Geometry: final body of the model. Coordinates: model frame, mm. Coordinates: 2 decimals unless noted, no trailing zeros. Write each loop counter-clockwise with the first axis right and the second up, starting at its lowest first coordinate (ties: lowest second). Pieces come first, ordered by that corner, then holes. Notation, with made-up numbers: (-2, 13.25) -> (9, 13.25) arc R17 cw to (9, 40.25) -> close; hole circle Ø9 at (-13, 76.25). An arc over 180 degrees is marked (long way). Answer as a JSON object with one key per item and string values. Group by question number.
```python
from build123d import *

# Parameters (mm, degrees)
F1_DEPTH = 1.7
F2_R     = 3
F3_W     = 62.5
F3_H     = 32
F4_DEPTH = 1.701
F5_R     = 5


with BuildPart() as f1:
    # F0 (on Top) → F1 (new body)
    with BuildSketch(Plane.XY):
        Polygon((100.0762677759, 54.24722471), (-84.9237322241, 54.24722471), (-84.9237322241, 39.24722471), (-72.9237322241, 39.24722471), (-72.9237322241, 36.24722471), (-72.9237322241, -37.75277529), (-72.9237322241, -40.75277529), (-84.9237322241, -40.75277529), (-84.9237322241, -55.75277529), (100.0762677759, -55.75277529), (100.0762677759, -40.75277529), (88.0762677759, -37.75277529), (88.0762677759, 36.24722471), (88.0762677759, 39.24722471), (100.0762677759, 39.24722471), align=None)
        Polygon((88.0762677759, 36.24722471), (100.0762677759, 39.24722471), (88.0762677759, 39.24722471), align=None)
        Polygon((-72.9237322241, 39.24722471), (-84.9237322241, 39.24722471), (-72.9237322241, 36.24722471), align=None)
        Polygon((-72.9237322241, -40.75277529), (-72.9237322241, -37.75277529), (-84.9237322241, -40.75277529), align=None)
    extrude(amount=F1_DEPTH)

    # F2
    f2_edges = [f1.edges().sort_by_distance(p)[0] for p in [
        (-72.923732, -37.752775, 0.85),
        (-72.923732, 36.247225, 0.85),
        (-84.923732, 39.247225, 0.85),
        (-84.923732, -40.752775, 0.85),
        (88.076268, 36.247225, 0.85),
        (100.076268, 39.247225, 0.85),
        (-84.923732, -55.752775, 0.85),
        (-84.923732, 54.247225, 0.85),
        (100.076268, 54.247225, 0.85),
        (100.076268, -55.752775, 0.85),
        (100.076268, -40.752775, 0.85),
        (88.076268, -37.752775, 0.85),
    ]]
    fillet(f2_edges, radius=F2_R)

    # F3 (on face) → F4 (cut, through all)
    with BuildSketch(Plane.XY.offset(1.7)):
        with Locations((-26.6737322241, 18.24722471)):
            Rectangle(F3_W, F3_H)
        with Locations((-26.6737322241, -19.75277529)):
            Rectangle(F3_W, F3_H)
        with Locations((41.8262677759, 18.24722471)):
            Rectangle(F3_W, F3_H)
        with Locations((41.8262677759, -19.75277529)):
            Rectangle(F3_W, F3_H)
    extrude(amount=-F4_DEPTH, mode=Mode.SUBTRACT)

    # F5
    f5_edges = [f1.edges().sort_by_distance(p)[0] for p in [
        (-57.923732, 34.247225, 0.85),
        (4.576268, 2.247225, 0.85),
        (73.076268, -35.752775, 0.85),
        (10.576268, -35.752775, 0.85),
        (10.576268, 2.247225, 0.85),
        (10.576268, -3.752775, 0.85),
        (10.576268, 34.247225, 0.85),
        (-57.923732, -3.752775, 0.85),
        (4.576268, -3.752775, 0.85),
        (73.076268, -3.752775, 0.85),
        (4.576268, -35.752775, 0.85),
        (-57.923732, -35.752775, 0.85),
        (4.576268, 34.247225, 0.85),
        (-57.923732, 2.247225, 0.85),
        (73.076268, 34.247225, 0.85),
        (73.076268, 2.247225, 0.85),
    ]]
    fillet(f5_edges, radius=F5_R)


solid = f1.part
```
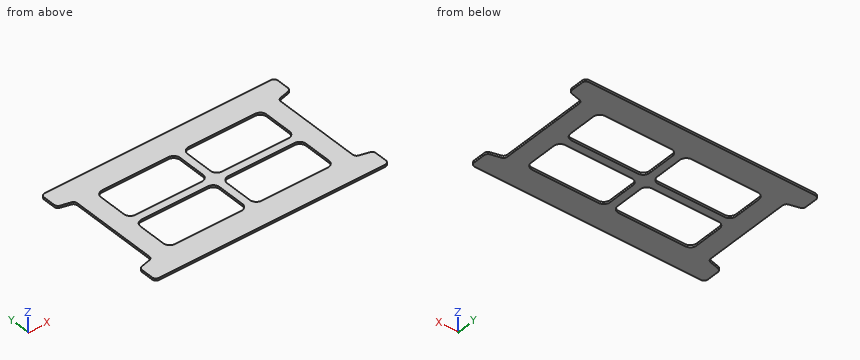
Item 1: Section A-A on x = 51. Output: boundary loops of the cut face in (y, z), then the cut area to 3 significant figures.
Item 2: Section C-C on z = 0.75. Give the number of separate pieces and of enclosed holes in the cut face, then the cut area to 3 significant figures.
Item 3: Section B-B on y = -17. Output: boundary loops of the cut face in (x, z), then the cut area to 3 significant figures.
Item 4: Contact query for flat-ended pins moving along their axis: pin 1 (0.8 mm diameter, centred on y = -15.5, z = 1, fed in from -X); pin 2 (0.8 mm diameter, centred on y = -24, z = 0.5, fed in from +X). Output: stop coordinate, or through.
Item 5: Ray query, L1, parallel to Y at x = 23.5, z = 0.7; L2, parallel to X at y = 29, z = 1; L3, parallel to Y at x = 13, z = 0.5. Return the intervals inside material, ascending. Write a range as [from, to].
Answer sheet:
{
 "1": {"outline": "(-55.75, 0) -> (-35.75, 0) -> (-35.75, 1.7) -> (-55.75, 1.7) -> close; (-3.75, 0) -> (2.25, 0) -> (2.25, 1.7) -> (-3.75, 1.7) -> close; (34.25, 0) -> (54.25, 0) -> (54.25, 1.7) -> (34.25, 1.7) -> close", "area": "78.2 mm^2"},
 "2": {"separate pieces": "1", "enclosed holes": "4", "area": "10,600 mm^2"},
 "3": {"outline": "(-72.92, 0) -> (-57.92, 0) -> (-57.92, 1.7) -> (-72.92, 1.7) -> close; (4.58, 0) -> (10.58, 0) -> (10.58, 1.7) -> (4.58, 1.7) -> close; (73.08, 0) -> (88.08, 0) -> (88.08, 1.7) -> (73.08, 1.7) -> close", "area": "61.2 mm^2"},
 "4": {"pin 1": "stops at x = -72.92", "pin 2": "stops at x = 88.08"},
 "5": {"L1": "y = [-55.75, -35.75], [-3.75, 2.25], [34.25, 54.25]", "L2": "x = [-72.92, -57.92], [4.58, 10.58], [73.08, 88.08]", "L3": "y = [-55.75, -35.04], [-4.47, 2.96], [33.53, 54.25]"}
}
